```python
from build123d import *

# Parameters (mm, degrees)
SKETCH004_W                     = 28
SKETCH004_H                     = 28
SKETCH004_R                     = 2
PAD004_DEPTH                    = 0.2
SKETCH005_W                     = 3.5
SKETCH005_H                     = 1.8
PAD005_DEPTH                    = 0.8
SKETCH005_LINEARPATTERN003_2_W  = 3.5
SKETCH005_LINEARPATTERN003_2_H  = 1.8
PAD005_LINEARPATTERN003_2_DEPTH = 0.8
SKETCH005_LINEARPATTERN003_3_W  = 3.5
SKETCH005_LINEARPATTERN003_3_H  = 1.8
PAD005_LINEARPATTERN003_3_DEPTH = 0.8
SKETCH005_LINEARPATTERN003_4_W  = 3.5
SKETCH005_LINEARPATTERN003_4_H  = 1.8
PAD005_LINEARPATTERN003_4_DEPTH = 0.8


with BuildPart() as part:
    # Sketch004 → Pad004 (new body)
    with BuildSketch(Plane.XY.offset(0.5)):
        Rectangle(SKETCH004_W, SKETCH004_H)
        with Locations((-7.9, 7.9)):
            Circle(SKETCH004_R, mode=Mode.SUBTRACT)
        with Locations((7.9, 7.9)):
            Circle(SKETCH004_R, mode=Mode.SUBTRACT)
        with Locations((7.9, -7.9)):
            Circle(SKETCH004_R, mode=Mode.SUBTRACT)
        with Locations((-7.9, -7.9)):
            Circle(SKETCH004_R, mode=Mode.SUBTRACT)
    extrude(amount=PAD004_DEPTH)

    # Sketch005 → Pad005 (join)
    with BuildSketch(Plane.XY.offset(-0.2)):
        with Locations((-12.85, -3.8)):
            Rectangle(SKETCH005_W, SKETCH005_H)
    pad005 = extrude(amount=PAD005_DEPTH)

    # Sketch005 LinearPattern003 2 → Pad005 LinearPattern003 2 (add)
    with BuildSketch(Plane(origin=(0, 2.5333333333, -0.2), x_dir=(1, 0, 0), z_dir=(0, 0, 1))):
        with Locations((-12.85, -3.8)):
            Rectangle(SKETCH005_LINEARPATTERN003_2_W, SKETCH005_LINEARPATTERN003_2_H)
    pad005_linearpattern003_2 = extrude(amount=PAD005_LINEARPATTERN003_2_DEPTH)

    # Sketch005 LinearPattern003 3 → Pad005 LinearPattern003 3 (add)
    with BuildSketch(Plane(origin=(0, 5.0666666667, -0.2), x_dir=(1, 0, 0), z_dir=(0, 0, 1))):
        with Locations((-12.85, -3.8)):
            Rectangle(SKETCH005_LINEARPATTERN003_3_W, SKETCH005_LINEARPATTERN003_3_H)
    pad005_linearpattern003_3 = extrude(amount=PAD005_LINEARPATTERN003_3_DEPTH)

    # Sketch005 LinearPattern003 4 → Pad005 LinearPattern003 4 (add)
    with BuildSketch(Plane(origin=(0, 7.6, -0.2), x_dir=(1, 0, 0), z_dir=(0, 0, 1))):
        with Locations((-12.85, -3.8)):
            Rectangle(SKETCH005_LINEARPATTERN003_4_W, SKETCH005_LINEARPATTERN003_4_H)
    pad005_linearpattern003_4 = extrude(amount=PAD005_LINEARPATTERN003_4_DEPTH)

    # Mirrored001: Pad005, Pad005 LinearPattern003 2, Pad005 LinearPattern003 3, Pad005 LinearPattern003 4 across YZ
    add(pad005.mirror(Plane.YZ))
    add(pad005_linearpattern003_2.mirror(Plane.YZ))
    add(pad005_linearpattern003_3.mirror(Plane.YZ))
    add(pad005_linearpattern003_4.mirror(Plane.YZ))


solid = part.part
```
The listing builds one solid part. Answer for the finished solid, in the listing's coordinates (mm). Coordinates: 2 decimals unless noted, no trailing zeros. Loops run counter-clockwise (first coordinate to the right, second up) from the corner with the lowest first, then second, coordinate; pieces in that order, holes last. Notation, with made-up numbers: (2, 39.5) -> (23, 39.5) arc R21 ccw to (23, 56.5) -> close; hole circle Ø5 at (8, 4.25). An arc over 180 degrees is marked (long way). Return JSON: item names as keys, results as strings. Group by question number.
(1) Find the intervals of material crossed by probe 1 along Y at (x, z) = (7.9, 0.65); probe 2 along Y at (x, z) = (-12.25, 0.3); probe 3 along X at (y, z) = (2, 0.3), in increasing order. Write a range as from..to.
(2) A cutting plane is placed at A-A on z = 0.3. Count the separate pieces of the cut face and the enclosed holes in it, and give its area (3 significant figures).
(3) A cutting plane is placed at D-D on x = -10.5. Write down the section's boundary in (y, z).
(4) Given pin 1 Ø10 at (x, y) = (2, 10.5) entering from -Z, flat-ended and moving along its own axis, determine where the tip first touches the part or whether it passes through.
(5) A cutting plane is placed at B-B on x = 7.9. Write down the section's boundary in (y, z).
The answers:
{
 "1": {"probe 1": "y = -14..-9.9, -5.9..5.9, 9.9..14", "probe 2": "y = -4.7..-2.9, -2.17..-0.37, 0.37..2.17, 2.9..4.7", "probe 3": "x = -14.6..-11.1, 11.1..14.6"},
 "2": {"separate pieces": "8", "enclosed holes": "0", "area": "50.4 mm^2"},
 "3": {"outline": "(-14, 0.5) -> (14, 0.5) -> (14, 0.7) -> (-14, 0.7) -> close"},
 "4": {"pin 1": "stops at z = 0.5"},
 "5": {"outline": "(-14, 0.5) -> (-9.9, 0.5) -> (-9.9, 0.7) -> (-14, 0.7) -> close; (-5.9, 0.5) -> (5.9, 0.5) -> (5.9, 0.7) -> (-5.9, 0.7) -> close; (9.9, 0.5) -> (14, 0.5) -> (14, 0.7) -> (9.9, 0.7) -> close"}
}
